Check sheet for the modelled part. Datum: model origin and axes. Units: mm. Face numbers are marked on the shaded views. Coordinates: 2 decimals unless noted, no trailing zeros. Write each loop counter-clockwise with the first axis right and the second up, starting at its lowest first coordinate (ties: lowest second). Pieces come first, ordered by that corner, then holes. Notation, with made-up numbers: M -15,80.25 L 31,80.25 A16 ccw 31,109.25 Z; hole C 87.25,20 d4. An arc over 180 degrees is marked long. Answer as CSV lines item,"result". Start each with the question number.
Q1. Mould release check, pull along Z, two halves, no side actions. Record for the marked faces 1 and 2: pulls with the +Z half, pulls with the -Z half, needs draft (parallel to the pull), parting line crosses it, or undercut.
Q2. Depth check by flat-ended pin: pin 1 Ø1.5 at (x, z) = (-77, 2) entering from +Y; pin 2 Ø1 at (x, z) = (-53.5, 2) entering from -Y; pin 3 Ø1.5 at (y, z) = (36.5, 1.5) entering from -X. Enter the tip coordinate at first touch or a pass-through.
Q3. Sectioned sample at C-C, the plane x = -30.5. Record the cut outline in (y, z), then the cut area to 3 significant figures.
Q4. Sectioned sample at A-A, the plane x = 0. Record the cut outline in (y, z), then the cut area to 3 significant figures.
Q5. Thickness scan on line 1 along Y through (x, z) = (48.5, 0.6); line 2 along Y through (x, z) = (-8.5, 0.9); line 3 along Y through (x, z) = (0, 2.1). Record the ranges inside material, lowest first. Write a range as from..to.
Q6. Sectioned sample at B-B, the plane z = 1.3. Count the separate pieces of the cut face and the enclosed holes in it, then the cut area to 3 significant figures.
Q7. Sectioned sample at D-D, the plane y = -42. Record the cut outline in (x, z).
Autodesk Inventor part; units mm, degrees
ref_plane "YZ Plane" through (0, 0, 0) normal (1, 0, 0) x (0, 1, 0)
ref_plane "XZ Plane" through (0, 0, 0) normal (0, 1, 0) x (-1, 0, 0)
ref_plane "XY Plane" through (0, 0, 0) normal (0, 0, 1) x (1, 0, 0)
sketch "Эскиз1" plane through (0, 0, 0) normal (0, 0, 1) x (1, 0, 0)
  line L0 (0, 53) -> (5, 53)
  line L1 (5, 53) -> (5, 50)
  line L2 (32.5, 53) -> (42.5, 53)
  line L3 (42.5, 53) -> (42.5, 50)
  line L4 (32.5, 50) -> (32.5, 53)
  line L5 (78, 30) -> (75, 30)
  line L6 (75, 20) -> (78, 20)
  line L7 (78, 20) -> (78, 30)
  line L8 (78, 5) -> (75, 5)
  line L9 (78, 0) -> (78, 5)
  line L10 (5, 50) -> (32.5, 50)
  line L11 (42.5, 50) -> (75, 50)
  line L12 (5, 50) -> (32.5, 50)
  line L13 (42.5, 50) -> (75, 50)
  line L14 (75, 50) -> (75, 30)
  line L15 (75, 20) -> (75, 5)
  line L16 (75, 50) -> (75, 30)
  line L17 (75, 20) -> (75, 5)
  line L18 (0, -53) -> (5, -53)
  line L19 (5, -53) -> (5, -50)
  line L20 (32.5, -53) -> (42.5, -53)
  line L21 (42.5, -53) -> (42.5, -50)
  line L22 (32.5, -50) -> (32.5, -53)
  line L23 (78, -30) -> (75, -30)
  line L24 (75, -20) -> (78, -20)
  line L25 (78, -20) -> (78, -30)
  line L26 (78, -5) -> (75, -5)
  line L27 (78, 0) -> (78, -5)
  line L28 (5, -50) -> (32.5, -50)
  line L29 (42.5, -50) -> (75, -50)
  line L30 (5, -50) -> (32.5, -50)
  line L31 (42.5, -50) -> (75, -50)
  line L32 (75, -50) -> (75, -30)
  line L33 (75, -20) -> (75, -5)
  line L34 (75, -50) -> (75, -30)
  line L35 (75, -20) -> (75, -5)
  line L36 (0, 53) -> (-5, 53)
  line L37 (-5, 53) -> (-5, 50)
  line L38 (-32.5, 53) -> (-42.5, 53)
  line L39 (-42.5, 53) -> (-42.5, 50)
  line L40 (-32.5, 50) -> (-32.5, 53)
  line L41 (-78, 30) -> (-75, 30)
  line L42 (-75, 20) -> (-78, 20)
  line L43 (-78, 20) -> (-78, 30)
  line L44 (-78, 5) -> (-75, 5)
  line L45 (-78, 0) -> (-78, 5)
  line L46 (-5, 50) -> (-32.5, 50)
  line L47 (-42.5, 50) -> (-75, 50)
  line L48 (-5, 50) -> (-32.5, 50)
  line L49 (-42.5, 50) -> (-75, 50)
  line L50 (-75, 50) -> (-75, 30)
  line L51 (-75, 20) -> (-75, 5)
  line L52 (-75, 50) -> (-75, 30)
  line L53 (-75, 20) -> (-75, 5)
  line L54 (-32.5, -53) -> (-42.5, -53)
  line L55 (-32.5, -50) -> (-32.5, -53)
  line L56 (-5, -50) -> (-32.5, -50)
  line L57 (-5, -50) -> (-32.5, -50)
  line L58 (-5, -53) -> (-5, -50)
  line L59 (0, -53) -> (-5, -53)
  line L60 (-42.5, -53) -> (-42.5, -50)
  line L61 (-42.5, -50) -> (-75, -50)
  line L62 (-42.5, -50) -> (-75, -50)
  line L63 (-75, -50) -> (-75, -30)
  line L64 (-75, -50) -> (-75, -30)
  line L65 (-78, -30) -> (-75, -30)
  line L66 (-75, -20) -> (-78, -20)
  line L67 (-78, -20) -> (-78, -30)
  line L68 (-75, -20) -> (-75, -5)
  line L69 (-75, -20) -> (-75, -5)
  line L70 (-78, -5) -> (-75, -5)
  line L71 (-78, 0) -> (-78, -5)
  circle A0 centre (23.5, 30) radius 1
  circle A1 centre (48.5, 30) radius 1
  circle A2 centre (23.5, -30) radius 1
  circle A3 centre (48.5, -30) radius 1
  circle A4 centre (-60, 24) radius 1.5
  circle A5 centre (-61, -24) radius 1.5
  circle A6 centre (-8.5, -19) radius 1.5
  circle A7 centre (-8.5, 8.5) radius 1.5
  circle A8 centre (0, 30) radius 7.5
  point P0 (37.5, 50)
  point P1 (75, 25)
  point P2 (37.5, -50)
  point P3 (75, -25)
  point P4 (-37.5, 50)
  point P5 (-37.5, -50)
  point P6 (36, 0)
  dimension "d48" = 15
extrude "Выдавливание3" add sketch "Эскиз1" along normal blind 3
sketch "Эскиз3" plane through (0, 0, 3) normal (0, 0, 1) x (1, 0, 0)
  line L0 (-75, 30) -> (-78, 30)
  line L1 (-42.5, 50) -> (-75, 50)
  line L2 (-78, 20) -> (-75, 20)
  line L3 (-75, 5) -> (-78, 5)
  line L4 (-75, -50) -> (-42.5, -50)
  point P0 (0, 0)
  dimension "d51" = 20
  dimension "d52" = 10
  dimension "d53" = 15
  dimension "d54" = 100
properties part number "крепления"
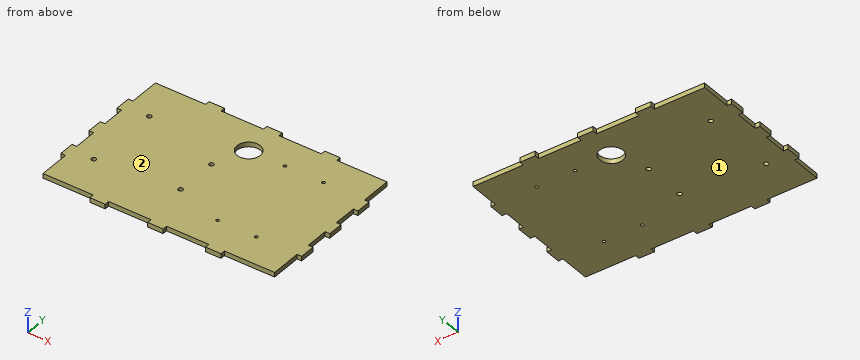
Output:
1,face 1,"pulls with the -Z half"
1,face 2,"pulls with the +Z half"
2,pin 1,"stops at y = 30"
2,pin 2,"stops at y = -50"
2,pin 3,"stops at x = -75"
3,outline,"M -50,0 L 50,0 L 50,3 L -50,3 Z"
3,area,"300 mm^2"
4,outline,"M -53,0 L 22.5,0 L 22.5,3 L -53,3 Z; M 37.5,0 L 53,0 L 53,3 L 37.5,3 Z"
4,area,"273 mm^2"
5,line 1,"y = -50..-31, -29..29, 31..50"
5,line 2,"y = -50..-20.5, -17.5..7, 10..50"
5,line 3,"y = -53..22.5, 37.5..53"
6,separate pieces,"1"
6,enclosed holes,"9"
6,area,"15,100 mm^2"
7,outline,"M -75,0 L 75,0 L 75,3 L -75,3 Z"
